Verification items for the finished model (mm, model axes). Face numbers are marked on the shaded views. A direction names the side the tool comes from. Give positions to 0.01 mm unless a question says otherwise; leave off trailing zeros. Loops run counter-clockwise (first coordinate to the right, second up) from the corner with the lowest first, then second, coordinate; pieces in that order, holes last. Notation, with made-up numbers: (42.25, 62) - (86.25, 62) arc R14 cw to (86.25, 78) - close; hole circle Ø9 at (-11.5, 70.25). An arc over 180 degrees is marked (long way). One line per question, with ' | ' between items. Start each with the question number.
1. Tool access check on the marked faces 1 and 2. Record the directions out of +Z, -Z, +X, -X, +Y, -Y that give a thin tool (end or side, any length) a straight path to the whole face; none if there is none.
2. Section check C-C, the plane x = 39.5. Enter the section's corners in (y, z) (3 decimals).
3. Section check B-B, the plane z = 47.8. Enter the section's corners in (x, y) (3 decimals), then the cut area to 3 significant figures.
4. Section check D-D, the plane z = 5.9. Enter the section's corners in (x, y) (3 decimals), then the cut area to 3 significant figures.
5. Section check A-A, the plane x = 6. Enter the section's corners in (y, z) (3 decimals), then the cut area to 3 significant figures.
6. Depth check by flat-ended pin: pin 1 Ø4 at (x, z) = (6, 7) entering from +Y; pin 2 Ø3 at (x, z) = (8.5, 14.4) entering from -Y; pin 3 Ø3 at (y, z) = (-3, 42.5) entering from +X. Enter the tip coordinate at first touch or a pass-through.
7. Thickness scan on line 1 along Z through (x, y) = (6, -8.2); line 2 along X through (y, z) = (-2.5, 14.5); line 3 along Z through (x, y) = (39.5, -2.05) (3 decimals). Record the ranges inside material, lowest first. Write a range as from..to.
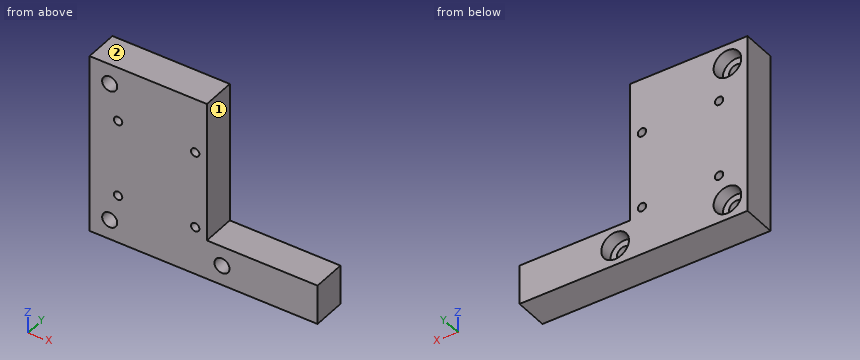
from build123d import *

# Parameters (mm, degrees)
SKETCH1_W                                           = 68
SKETCH1_H                                           = 53.8
BOSS_EXTRUDE1_DEPTH                                 = 10
SKETCH2_W                                           = 33
SKETCH2_H                                           = 42
CUT_EXTRUDE1_DEPTH                                  = 11
F_2_CLEARANCE_HOLE1_D                               = 2.5
F_2_CLEARANCE_HOLE1_DEPTH                           = 10
CBORE_FOR_8_BINDING_HEAD_MACHINE_SCREW1_D           = 4.5
CBORE_FOR_8_BINDING_HEAD_MACHINE_SCREW1_DEPTH       = 10
CBORE_FOR_8_BINDING_HEAD_MACHINE_SCREW1_CBORE_D     = 8.25
CBORE_FOR_8_BINDING_HEAD_MACHINE_SCREW1_CBORE_DEPTH = 4


with BuildPart() as part:
    # Sketch1 → Boss-Extrude1 (new body)
    with BuildSketch(Plane(origin=(0, 0, 0), x_dir=(1, 0, 0), z_dir=(0, 1, 0))):
        with Locations((34, -26.9)):
            Rectangle(SKETCH1_W, SKETCH1_H)
    extrude(amount=-BOSS_EXTRUDE1_DEPTH)

    # Sketch2 → Cut-Extrude1 (cut, through all)
    with BuildSketch(Plane.XZ.offset(10)):
        with Locations((51.5, 32.8)):
            Rectangle(SKETCH2_W, SKETCH2_H)
    extrude(amount=-CUT_EXTRUDE1_DEPTH, mode=Mode.SUBTRACT)

    # #2 Clearance Hole1
    with Locations(Plane(origin=(0, -10, 0), x_dir=(-1, 0, 0), z_dir=(0, -1, 0))):
        with Locations((-31.502183488, -14.402425), (-31.5, -37.404608488), (-8.497816512, -37.402425), (-8.5, -14.400241512)):
            Hole(F_2_CLEARANCE_HOLE1_D / 2, depth=F_2_CLEARANCE_HOLE1_DEPTH)

    # CBORE for #8 Binding Head Machine Screw1
    with Locations(Plane(origin=(0, 0, 0), x_dir=(1, 0, 0), z_dir=(0, 1, 0))):
        with Locations((6, -47.8), (6, -5.9), (39.5, -5.9)):
            CounterBoreHole(CBORE_FOR_8_BINDING_HEAD_MACHINE_SCREW1_D / 2, CBORE_FOR_8_BINDING_HEAD_MACHINE_SCREW1_CBORE_D / 2, CBORE_FOR_8_BINDING_HEAD_MACHINE_SCREW1_CBORE_DEPTH, depth=CBORE_FOR_8_BINDING_HEAD_MACHINE_SCREW1_DEPTH)


solid = part.part
Results list:
1) face 1: +Z, +X, +Y, -Y | face 2: +Z, +X, -X, +Y, -Y
2) outline: (-10, 0) - (0, 0) - (0, 1.775) - (-4, 1.775) - (-4, 3.65) - (-10, 3.65) - close; (-10, 8.15) - (-4, 8.15) - (-4, 10.025) - (0, 10.025) - (0, 11.8) - (-10, 11.8) - close
3) outline: (0, -10) - (3.75, -10) - (3.75, -4) - (1.875, -4) - (1.875, 0) - (0, 0) - close; (8.25, -10) - (35, -10) - (35, 0) - (10.125, 0) - (10.125, -4) - (8.25, -4) - close | area: 290 mm²
4) outline: (0, -10) - (3.75, -10) - (3.75, -4) - (1.875, -4) - (1.875, 0) - (0, 0) - close; (8.25, -10) - (37.25, -10) - (37.25, -4) - (35.375, -4) - (35.375, 0) - (10.125, 0) - (10.125, -4) - (8.25, -4) - close; (41.75, -10) - (68, -10) - (68, 0) - (43.625, 0) - (43.625, -4) - (41.75, -4) - close | area: 560 mm²
5) outline: (-10, 0) - (0, 0) - (0, 1.775) - (-4, 1.775) - (-4, 3.65) - (-10, 3.65) - close; (-10, 8.15) - (-4, 8.15) - (-4, 10.025) - (0, 10.025) - (0, 43.675) - (-4, 43.675) - (-4, 45.55) - (-10, 45.55) - close; (-10, 50.05) - (-4, 50.05) - (-4, 51.925) - (0, 51.925) - (0, 53.8) - (-10, 53.8) - close | area: 418 mm²
6) pin 1: y = -4 | pin 2: y = -10 | pin 3: x = 35
7) line 1: 0..3.65, 8.15..45.55, 50.05..53.8 | line 2: 0..7.25, 9.75..30.26, 32.75..35 | line 3: 0..1.775, 10.025..11.8
